Design review of the part built by this model. Coordinates are the model's own, in mm. A direction names the side the tool comes from. Coordinates: 2 decimals unless noted, no trailing zeros. Loops run counter-clockwise (first coordinate to the right, second up) from the corner with the lowest first, then second, coordinate; pieces in that order, holes last. Notation, with made-up numbers: M 48.25,-25 L 105.25,-25 A15 cw 105.25,2 Z; hole C 51,36 d10. An arc over 180 degrees is marked long. Answer as a JSON object with one key per item and string values. Group by question number.
1. Draft analysis for pull direction Y (two halves, no side actions). For faces 1 (the flat face through (21.15, -17, 0)), 2 (the flat face through (0, -58, 0)), 3 (the flat face through (0, 0, 0)), state which applies: +Y half, -Y half, draft (parallel to the pull), parting line (faces both ways), or undercut.
2. Insertion check: pin 1 (5 mm diameter, centred on x = -15.5, y = -23.5, fed in from -Z); pin 2 (1.5 mm diameter, centred on x = -2.5, z = -12, fed in from -Y). Each pin has a flat end and moves straight along its axis. Give the tip position at first contact, or say it passes through.
3. Machinability: for faces 4 (the cylindrical face through (18.14, -17.24, -18.3)), 5 (the flat face through (0, -36, -4)), which of the approach directions +Z, -Z, +X, -X, +Y, -Y give a long, thin tool a straight path to every point of the face, cutting with its end or side? Answer none if there is none.
4. Consider section A-A (y = -31). State the section outline as (x, z) points, then the cut area to 3 significant figures.
5. To check wall thickness, follow probe 1 along X at (y, z) = (-17.5, 15.5); probe 2 along X at (y, z) = (-13, 15). State the ranges of each line that lie inside material, in increasing order.
from build123d import *

# Parameters (mm, degrees)
F0_W     = 42.3
F0_H     = 42.3
F1_DEPTH = 34
F2_R     = 3
F3_DEPTH = 24
F5_DEPTH = 58.001
F6_R     = 11
F7_DEPTH = 2
F8_R     = 10
F9_R     = 1.99999


# Not quite as in the source:
# - a fillet or chamfer is up to 0.001 mm smaller than in the source, because OpenCascade refuses the exact size


with BuildPart() as f1:
    # F0 (on Front) → F1 (new body)
    with BuildSketch(Plane.XZ):
        Rectangle(F0_W, F0_H)
    extrude(amount=F1_DEPTH)

    # F2 (on face) → F3 (join)
    with BuildSketch(Plane.XZ.offset(34)):
        Circle(F2_R)
    extrude(amount=F3_DEPTH)

    # F4 (on face) → F5 (cut, through all)
    with BuildSketch(Plane(origin=(0, 0, 0), x_dir=(-1, 0, 0), z_dir=(0, 1, 0))):
        with BuildLine():
            Line((-15.5, 14.5), (-15.5, 15.5))
            Line((-15.5, 15.5), (-14.5, 15.5))
            ThreePointArc((-14.5, 15.5), (-16.2071067812, 16.2071067812), (-15.5, 14.5))
        make_face()
        with BuildLine():
            ThreePointArc((16.5, 15.5), (15.5, 16.5), (14.5, 15.5))
            Line((14.5, 15.5), (15.5, 15.5))
            Line((15.5, 15.5), (15.5, 14.5))
            ThreePointArc((15.5, 14.5), (16.2071067812, 14.7928932188), (16.5, 15.5))
        make_face()
        with BuildLine():
            Line((-15.5, -15.5), (-15.5, -14.5))
            ThreePointArc((-15.5, -14.5), (-16.2071067812, -16.2071067812), (-14.5, -15.5))
            Line((-14.5, -15.5), (-15.5, -15.5))
        make_face()
        with BuildLine():
            ThreePointArc((16.5, -15.5), (16.2071067812, -14.7928932188), (15.5, -14.5))
            Line((15.5, -14.5), (15.5, -15.5))
            Line((15.5, -15.5), (14.5, -15.5))
            ThreePointArc((14.5, -15.5), (15.5, -16.5), (16.5, -15.5))
        make_face()
        with BuildLine():
            Line((15.5, 15.5), (14.5, 15.5))
            ThreePointArc((14.5, 15.5), (14.7928932188, 14.7928932188), (15.5, 14.5))
            Line((15.5, 14.5), (15.5, 15.5))
        make_face()
        with BuildLine():
            Line((-14.5, 15.5), (-15.5, 15.5))
            Line((-15.5, 15.5), (-15.5, 14.5))
            ThreePointArc((-15.5, 14.5), (-14.7928932188, 14.7928932188), (-14.5, 15.5))
        make_face()
        with BuildLine():
            ThreePointArc((-14.5, -15.5), (-14.7928932188, -14.7928932188), (-15.5, -14.5))
            Line((-15.5, -14.5), (-15.5, -15.5))
            Line((-15.5, -15.5), (-14.5, -15.5))
        make_face()
        with BuildLine():
            Line((15.5, -15.5), (15.5, -14.5))
            ThreePointArc((15.5, -14.5), (14.7928932188, -14.7928932188), (14.5, -15.5))
            Line((14.5, -15.5), (15.5, -15.5))
        make_face()
    extrude(amount=-F5_DEPTH, mode=Mode.SUBTRACT)

    # F6 (on face) → F7 (join)
    with BuildSketch(Plane.XZ.offset(34)):
        Circle(F6_R)
    extrude(amount=F7_DEPTH)

    # F8
    f8_edges = [f1.edges().sort_by_distance(p)[0] for p in [
        (21.15, -17, 21.15),
        (-21.15, -17, 21.15),
        (21.15, -17, -21.15),
        (-21.15, -17, -21.15),
    ]]
    fillet(f8_edges, radius=F8_R)

    # F9 (radius 2 in the source; OpenCascade refuses exactly that, so slightly less here)
    f9_edges = [f1.edges().sort_by_distance(p)[0] for p in [
        (-11, -36, 0),
    ]]
    fillet(f9_edges, radius=F9_R)


solid = f1.part
Findings below:
{
 "1": {"face 1": "draft", "face 2": "-Y half", "face 3": "+Y half"},
 "2": {"pin 1": "stops at z = -20.98", "pin 2": "stops at y = -34"},
 "3": {"face 4": "-Z, +X, +Y, -Y", "face 5": "-Y"},
 "4": {"outline": "M -21.15,-11.15 A10 ccw -11.15,-21.15 L 11.15,-21.15 A10 ccw 21.15,-11.15 L 21.15,11.15 A10 ccw 11.15,21.15 L -11.15,21.15 A10 ccw -21.15,11.15 Z; hole C -15.5,-15.5 d2; hole C -15.5,15.5 d2; hole C 15.5,-15.5 d2; hole C 15.5,15.5 d2", "area": "1,690 mm^2"},
 "5": {"probe 1": "x = -20.15 to -16.5, -14.5 to 14.5, 16.5 to 20.15", "probe 2": "x = -20.38 to -16.37, -14.63 to 14.63, 16.37 to 20.38"}
}
